Input: part model. Units: mm. Frame: model coordinates. A direction names the side the tool comes from. Coordinates: 2 decimals unless noted, no trailing zeros. Write each loop counter-clockwise with the first axis right and the second up, starting at its lowest first coordinate (ties: lowest second). Pieces come first, ordered by that corner, then holes. Notation, with made-up numbers: (0, 4.25) - (40, 4.25) arc R24 cw to (40, 25.25) - close; hole circle Ø2 at (9.5, 78.25). An arc over 180 degrees is marked (long way). Put each result on its own line as item: value. Start each with the question number.
1. Cut plane B-B, the plane y = 30.5. Return loops of the section in (x, z).
2. Line query: line 1 (Y direction, x = -5.5, z = 8); line 2 (Z direction, x = 1, y = 31); line 3 (Z direction, x = -5, y = 21). Output: solid intervals per line, ascending.
3. Pin query (flat end, axial travel): pin 1 (8 mm diameter, centred on x = -6, y = 7, fed in from -Z); pin 2 (2 mm diameter, centred on x = 0, z = 6, fed in from -Y); pin 3 (8 mm diameter, centred on y = 14, z = -10, fed in from -X); pin 4 (8 mm diameter, centred on x = -6.5, z = 8, fed in from +Y). Return the tip coordinate at first contact, or that it passes through.
4. Cut plane A-A, the plane y = 23.5. Return loops of the section in (x, z).
5. Access query for faces 1 (the flat face through (-11.2, 3.175, 4.6)), 2 (the cylindrical face through (-5.86, 1.61, 11.267)). Directions: +Z, -Z, +X, -X, +Y, -Y. A direction counts if a zero-diameter tool reaches every point of the face in a straight line with its end or side. Return the directions, or none.
from build123d import *


with BuildPart() as part:
    # Sketch1 → Revolve1 (revolve)
    with BuildSketch(Plane.XY, mode=Mode.PRIVATE) as revolve1_sk:
        with BuildLine():
            Line((0, 0), (12.7, 0))
            Line((12.7, 0), (12.7, 3.175))
            Line((12.7, 3.175), (11.938, 3.175))
            ThreePointArc((11.938, 3.175), (11.460765371, 7.391187926), (10.16, 11.43))
            ThreePointArc((10.16, 11.43), (11.43, 12.7), (10.16, 13.97))
            ThreePointArc((10.16, 13.97), (7.700355765, 18.177295328), (6.35, 22.86))
            ThreePointArc((6.35, 22.86), (7.62, 24.13), (6.35, 25.4))
            ThreePointArc((6.35, 25.4), (7.099515829, 33.712257914), (0, 38.1))
            Line((0, 38.1), (0, 0))
        make_face()
    revolve(revolve1_sk.sketch.rotate(Axis((0, 38.1, 0), (0, -1, 0)), 180), axis=Axis((0, 38.1, 0), (0, -1, 0)))


solid = part.part
Report:
1. outline: circle Ø15.86 at (0, 0)
2. line 1: y = 0 to 14.58
2. line 2: z = -7.83 to 7.83
2. line 3: z = -4.51 to 4.51
3. pin 1: stops at z = -11.75
3. pin 2: stops at y = 0
3. pin 3: stops at x = -9.61
3. pin 4: stops at y = 34.98
4. outline: circle Ø14.91 at (0, 0)
5. face 1: +Y
5. face 2: +Y, -Y
